Geometry: see drawing. Coordinates: mm, zero at the bounding-box minimum. A direction names the side the tool comes from. Give positions to 0.01 mm unless a question says otherwise; leave off trailing zeros. Write each loop counter-clockwise with the first axis right and the second up, starting at its lowest first coordinate (ties: lowest second). Pieces come first, ordered by that corner, then holes. Notation, with made-up numbers: (59, 11.5) -> (110, 11.5) arc R14 ccw to (110, 37.5) -> close; hole circle Ø8 at (60, 67). An arc over 180 degrees is marked (long way). Use one line per item in the form item = value. Start each with the question number.
(1) Cut plane C-C, the plane z = 2. Output: boundary loops of the cut face in (x, y), and give its area (3 significant figures).
(2) Set-up query: the marked faces 5, 6 and 7. Return all of +Z, -Z, +X, -X, +Y, -Y with unobstructed straight access to the full face (end or side cutting, diameter ignored); none if empty.
(3) Cut plane A-A, the plane z = 5.5. Output: boundary loops of the cut face in (x, y), and give its area (3 significant figures).
(4) First-contact query: P1, Ø3, axis at x = 9.5, z = 5, coming from the -Y side; P2, Ø0.8, axis at y = 0.5, z = 8, coming from the +X side; P3, Ø0.8, axis at y = 0.5, z = 5.5, coming from the -X side. Flat tips, straight axial feed; report the tip coordinate or a pass-through.
(5) Cut plane D-D, the plane y = 0.2. Output: boundary loops of the cut face in (x, z), and give its area (3 significant figures).
(6) Draft query along X for the marked faces 1, 2, 3 and 4. Return one class per face: pulls with the +X half, pulls with the -X half, needs draft (parallel to the pull), parting line crosses it, or undercut.
(7) Cut plane B-B, the plane x = 6.75. Output: boundary loops of the cut face in (y, z), and give its area (3 significant figures).
(8) Material intervals for line 1 along X through (y, z) = (0.9, 5.5); line 2 along Y through (x, z) = (2.25, 9); line 3 along Y through (x, z) = (8.75, 4), sorted ascending. Write a range as from..to.
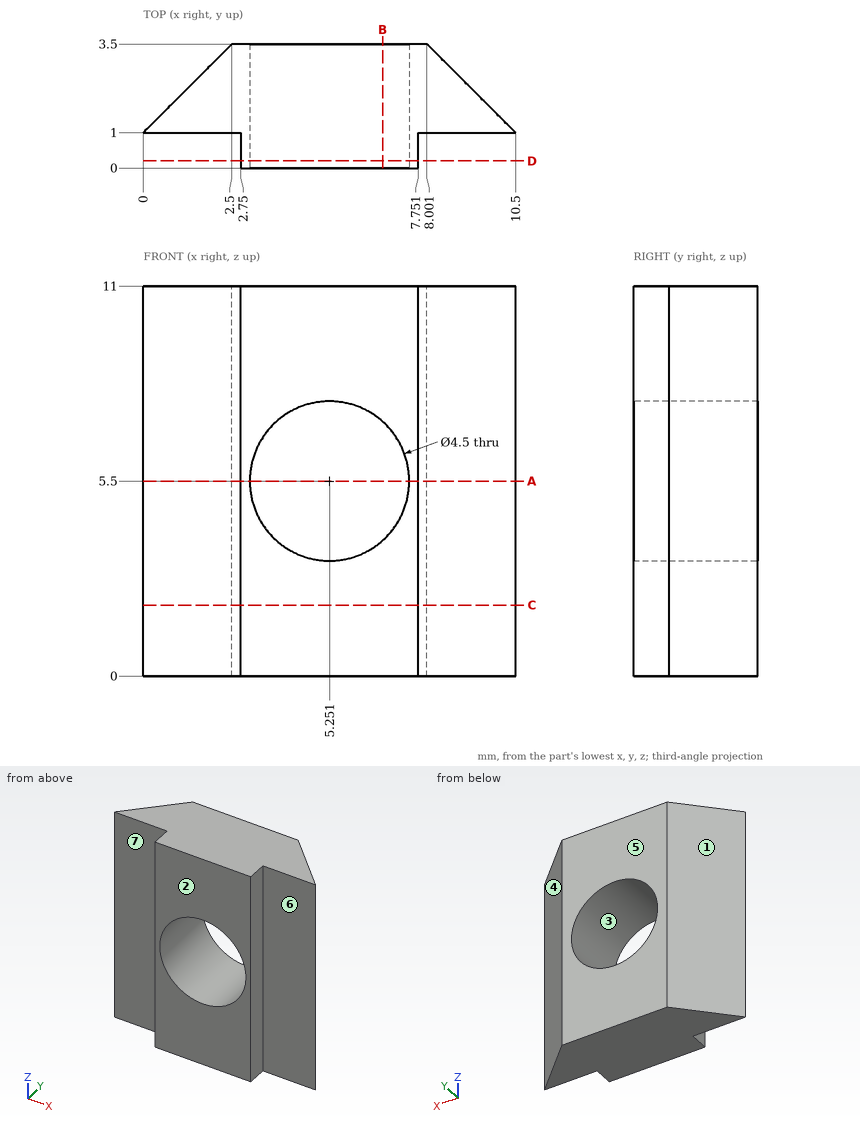
Geometry says:
q1.outline = (0, 1) -> (2.75, 1) -> (2.75, 0) -> (7.75, 0) -> (7.75, 1) -> (10.5, 1) -> (8, 3.5) -> (2.5, 3.5) -> close
q1.area = 25.0 mm^2
q2.face_5 = +Z, -Z, +X, -X, +Y
q2.face_6 = +Z, -Z, +X, -Y
q2.face_7 = +Z, -Z, -X, -Y
q3.outline = (0, 1) -> (2.75, 1) -> (2.75, 0) -> (3, 0) -> (3, 3.5) -> (2.5, 3.5) -> close; (7.5, 0) -> (7.75, 0) -> (7.75, 1) -> (10.5, 1) -> (8, 3.5) -> (7.5, 3.5) -> close
q3.area = 9.25 mm^2
q4.P1 = 1
q4.P2 = 7.75
q4.P3 = 2.75
q5.outline = (2.75, 0) -> (7.75, 0) -> (7.75, 11) -> (2.75, 11) -> close; hole circle Ø4.5 at (5.25, 5.5)
q5.area = 39.1 mm^2
q6.face_1 = pulls with the -X half
q6.face_2 = needs draft
q6.face_3 = undercut
q6.face_4 = pulls with the +X half
q7.outline = (0, 0) -> (3.5, 0) -> (3.5, 3.82) -> (0, 3.82) -> close; (0, 7.18) -> (3.5, 7.18) -> (3.5, 11) -> (0, 11) -> close
q7.area = 26.8 mm^2
q8.line_1 = 2.75..3, 7.5..7.75
q8.line_2 = 1..3.25
q8.line_3 = 1..2.75
